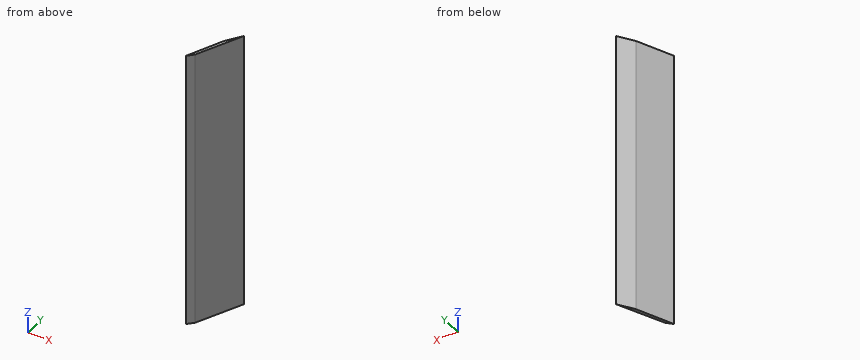
Autodesk Inventor part; units mm, degrees
ref_plane "YZ Plane" through (0, 0, 0) normal (1, 0, 0) x (0, 1, 0)
ref_plane "XZ Plane" through (0, 0, 0) normal (0, 1, 0) x (-1, 0, 0)
ref_plane "XY Plane" through (0, 0, 0) normal (0, 0, 1) x (1, 0, 0)
sketch "Sketch1" plane through (0, 0, 0) normal (0, 0, 1) x (1, 0, 0)
  line L0 (0, 57.4166) -> (-5, 46.6664)
  line L1 (-5, 42.7444) -> (-5, 46.6664)
  line L2 (-5, 42.7444) -> (-29.7, 18.0444)
  line L3 (-29.7, 18.0444) -> (-29.7, -5.3095)
  arc A0 (-5, 0) -> (-29.7, -5.3095) centre (-13.6, -20.1) ccw
  line L4 (0, 0) -> (-5, 0)
  line L5 (0, 0) -> (0, 57.4166)
  circle A1 centre (-13.6, -20.1) radius 16.1
  line L6 (2.5, -20.1) -> (2.5, 68.8205)
  line L7 (-13.6, -36.2) -> (-13.6, 63.8)
  line L8 (-13.6, 63.8) -> (7.5508, 63.8)
  line L9 (-5, 46.6664) -> (2.5, 62.7917)
  line L10 (2.5, 62.7917) -> (-1.25, 57.4166)
  line L11 (-1.25, 57.4166) -> (-6.961, 44.7054)
  line L12 (-6.961, 44.7054) -> (-5, 46.6664)
  dimension "d0" = 100
extrude "Extrusion1" add sketch "Sketch1" against normal blind 100 contours L0 L12 L11 L10 L9
ref_plane "Work Plane1" through (-5, 15.8, -50) normal (-1, 0, 0) x (0, 0, 1)
properties part number "nóż"
For this review, take the finished solid that the model builds, in its own axes (mm). Coordinates: 2 decimals unless noted, no trailing zeros. Write each loop counter-clockwise with the first axis right and the second up, starting at its lowest first coordinate (ties: lowest second). Pieces come first, ordered by that corner, then holes.
(1) Wall thickness on probe 1 along X at (y, z) = (45.5, -50); probe 2 along Y at (x, z) = (-3.75, -78); probe 3 along Y at (x, z) = (-1.5, -80): over which ranges is each line inside the solid? List them lowest first.
(2) Add section B-B on y = 56. Give the boundary of the cut face in (x, z).
(3) Add section A-A on z = -38.5. Give the boundary of the cut face in (x, y).
(4) For pin 1 Ø3 at (x, z) = (-2.5, -59) entering from -Y; pin 2 Ø5 at (x, z) = (-3, -69.5) entering from +Y; pin 3 Ø2 at (y, z) = (53.5, -32) entering from +X; pin 4 Ø2 at (x, y) = (-3.5, 59) entering from +Z, all flat-tipped, find the tip position at first contact; note any pin that passes through.
Answer sheet:
1. probe 1: x = -6.6 to -6.17
1. probe 2: y = 49.35 to 51.85
1. probe 3: y = 54.19 to 56.86
2. outline: (-1.89, -100) - (-0.66, -100) - (-0.66, 0) - (-1.89, 0) - close
3. outline: (-6.96, 44.71) - (-5, 46.67) - (2.5, 62.79) - (-1.25, 57.42) - close
4. pin 1: stops at y = 48.82
4. pin 2: stops at y = 58.49
4. pin 3: stops at x = -1.36
4. pin 4: passes through
